Can you work these out from the drawing? Everything is in mm from the part's minimum corner. A direction names the side the tool comes from. Give positions to 0.01 mm unless a question says otherwise; leave off trailing zeros. Loops run counter-clockwise (first coordinate to the right, second up) from the corner with the lowest first, then second, coordinate; pieces in that order, holes last.
Q1. I need wall thicknesses on line 1 (Y direction, x = 23.5, z = 7.4); line 2 (Y direction, x = 0.55, z = 3); line 3 (X direction, y = 11.75, z = 4.5). Which ranges of each line are inside material? Lowest first, please.
Q2. Will these pins go through, and if not, where does the flat tip stop? P1, Ø10, axis at x = 13, y = 5, coming from the -Z side; P2, Ø2, axis at y = 26, z = 3, coming from the +X side.
Q3. If we section it at B-B (z = 3): Please give me the cut outline in (x, y).
Q4. If we section it at A-A (x = 8.5): Please give me the cut outline in (y, z), plus the area to 3 significant figures.
Q5. For the marked faces 1 and 2, which set-ups out of +Z, -Z, +X, -X, +Y, -Y let a thin tool reach every point of the face, with its end or its side?
Q6. We'd pull the mould along X, two halves only. Please class the marked faces 3, 4, 5 and 6: +X half, -X half, draft (parallel to the pull), parting line (faces both ways), or undercut.
Q7. If we section it at C-C (y = 16): Please give me the cut outline in (x, z).
Q8. If we section it at D-D (y = 26): Please give me the cut outline in (x, z), plus the area to 3 significant figures.
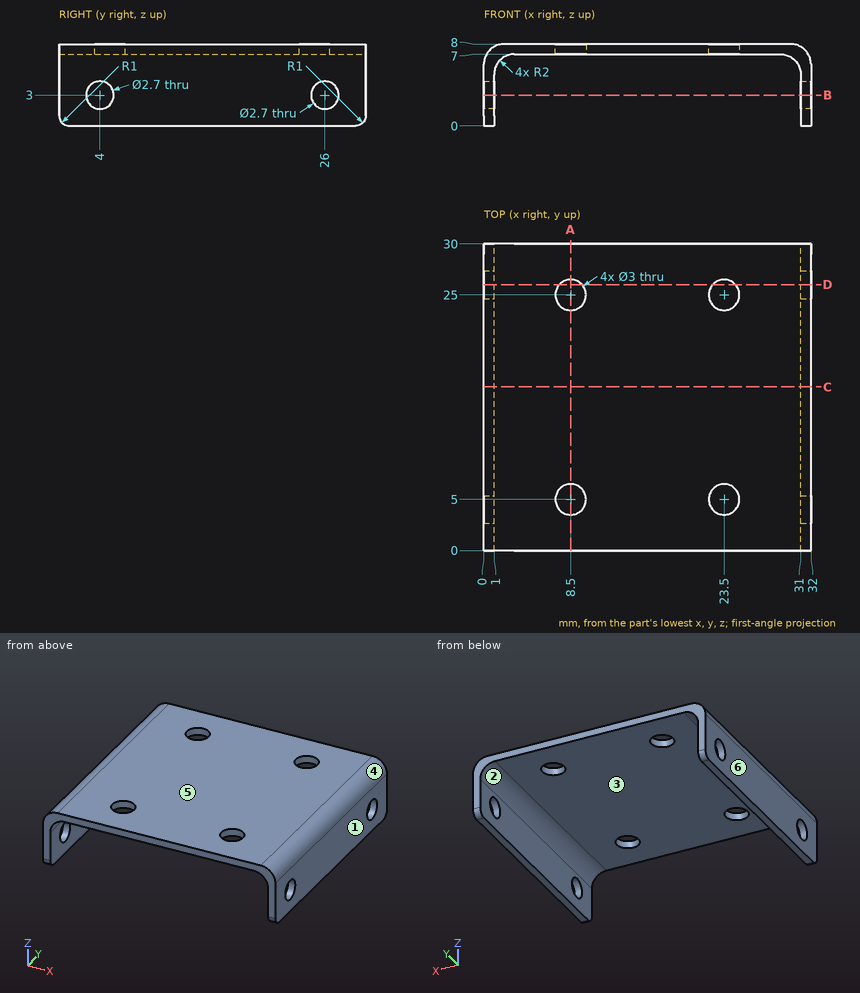
Check sheet entries:
1. line 1: y = 0 to 3.5, 6.5 to 23.5, 26.5 to 30
1. line 2: y = 0 to 2.65, 5.35 to 24.65, 27.35 to 30
1. line 3: x = 0 to 1, 31 to 32
2. P1: stops at z = 7
2. P2: passes through
3. outline: (0, 0) - (1, 0) - (1, 2.65) - (0, 2.65) - close; (0, 5.35) - (1, 5.35) - (1, 24.65) - (0, 24.65) - close; (0, 27.35) - (1, 27.35) - (1, 30) - (0, 30) - close; (31, 0) - (32, 0) - (32, 2.65) - (31, 2.65) - close; (31, 5.35) - (32, 5.35) - (32, 24.65) - (31, 24.65) - close; (31, 27.35) - (32, 27.35) - (32, 30) - (31, 30) - close
4. outline: (0, 7) - (3.5, 7) - (3.5, 8) - (0, 8) - close; (6.5, 7) - (23.5, 7) - (23.5, 8) - (6.5, 8) - close; (26.5, 7) - (30, 7) - (30, 8) - (26.5, 8) - close
4. area: 24.0 mm2
5. face 1: +Z, -Z, +X, +Y, -Y
5. face 2: -Z, +Y, -Y
6. face 3: undercut
6. face 4: +X half
6. face 5: draft
6. face 6: -X half
7. outline: (0, 0) - (1, 0) - (1, 5) arc R2 cw to (3, 7) - (29, 7) arc R2 cw to (31, 5) - (31, 0) - (32, 0) - (32, 6) arc R2 ccw to (30, 8) - (2, 8) arc R2 ccw to (0, 6) - close
8. outline: (0, 0) - (1, 0) - (1, 1.65) - (0, 1.65) - close; (0, 4.35) - (1, 4.35) - (1, 5) arc R2 cw to (3, 7) - (7.38, 7) - (7.38, 8) - (2, 8) arc R2 ccw to (0, 6) - close; (9.62, 7) - (22.38, 7) - (22.38, 8) - (9.62, 8) - close; (24.62, 7) - (29, 7) arc R2 cw to (31, 5) - (31, 4.35) - (32, 4.35) - (32, 6) arc R2 ccw to (30, 8) - (24.62, 8) - close; (31, 0) - (32, 0) - (32, 1.65) - (31, 1.65) - close
8. area: 36.1 mm2
